The model under review builds one solid part; all positions refer to its coordinate system, in mm. Round coordinates to 2 decimals unless told otherwise and drop trailing zeros. Order: outer loops, then holes, each group sorted by start corner. A loop starts at its lowest first (then second) coordinate and runs counter-clockwise, first axis right, second up. Notation, with made-up numbers: M 59,-8 L 113,-8 A16 ccw 113,18 Z; hole C 73,-29 d3. An arc over 180 degrees is marked long. Answer as a JSON object with one key per item and string values. Group by question number.
1. Add section C-C on y = 1. Give the number of separate pieces and of enclosed holes in the cut face, and give its area (3 significant figures).
2. Add section A-A on z = 0. State the section outline as (x, y) points, and give its area (3 significant figures).
3. Mouldability with a two-part tool opening along X and no side actions: class faces 1 (the face through (9.174, 0.986, 15.343)), 2 (the face through (-0.3, 0, 7.8)), 3 (the face through (-24.14, 1.01, -9.89)) as released by +X, released by -X, zero draft, split by the parting line, or undercut.
4. Add section B-B on x = 0. State the section outline as (y, z) points.
5. Add section D-D on z = 9.5. State the section outline as (x, y) points.
6. Clearance check with flat-ended pins moving along their axes: P1, Ø4, axis at x = 17.87, z = -4.79, coming from the +Y side; P2, Ø2.5, axis at x = -17.87, z = -4.79, coming from the +Y side. State where each tip first meets the part, or that it passes through.
7. To check wall thickness, follow probe 1 along Z at (x, y) = (10.5, 1.1); probe 2 along X at (y, z) = (1.15, -4.75); probe 3 along X at (y, z) = (1.5, -4). State the ranges of each line that lie inside material, in increasing order. Write a range as [from, to].
```python
from build123d import *

# Parameters (mm, degrees)
SKETCH_2_W      = 50
SKETCH_2_H      = 30.788152334
SKETCH_2_R      = 6.75
SKETCH_2_R_2    = 1.45
EXTRUDE_1_DEPTH = 2
FILLET_2_R      = 3


with BuildPart() as part:
    # 草图2 → 凸台-拉伸1 (new body)
    with BuildSketch(Plane(origin=(0, 0, 0), x_dir=(1, 0, 0), z_dir=(0, 1, 0))):
        with Locations((0, -4.605923833)):
            Rectangle(SKETCH_2_W, SKETCH_2_H)
        with Locations(Location((0, 0, 0), (0, 0, 270))):
            Circle(SKETCH_2_R, mode=Mode.SUBTRACT)
        with Locations(Location((-8.227241336, 4.75, 0), (0, 0, 270))):
            Circle(SKETCH_2_R_2, mode=Mode.SUBTRACT)
        with Locations(Location((0, -9.5, 0), (0, 0, 270))):
            Circle(SKETCH_2_R_2, mode=Mode.SUBTRACT)
        with Locations(Location((8.227241336, 4.75, 0), (0, 0, 90))):
            Circle(SKETCH_2_R_2, mode=Mode.SUBTRACT)
        with Locations(Location((-10.611164072, -15.154312819, 0), (0, 0, 270))):
            Circle(SKETCH_2_R_2, mode=Mode.SUBTRACT)
        with Locations(Location((-17.869627786, 4.788152334, 0), (0, 0, 270))):
            Circle(SKETCH_2_R_2, mode=Mode.SUBTRACT)
        with Locations(Location((10.611164072, -15.154312819, 0), (0, 0, 90))):
            Circle(SKETCH_2_R_2, mode=Mode.SUBTRACT)
        with Locations(Location((17.869627786, 4.788152334, 0), (0, 0, 90))):
            Circle(SKETCH_2_R_2, mode=Mode.SUBTRACT)
    extrude(amount=EXTRUDE_1_DEPTH)

    # 圆角2
    fillet_2_edges = [part.edges().sort_by_distance(p)[0] for p in [
        (25, 1, 20),
        (-25, 1, 20),
        (-25, 1, -10.788152334),
        (25, 1, -10.788152334),
    ]]
    fillet(fillet_2_edges, radius=FILLET_2_R)


solid = part.part
```
Recorded:
{
 "1": {"separate pieces": "1", "enclosed holes": "8", "area": "1,340 mm²"},
 "2": {"outline": "M -25,0 L -6.75,0 L -6.75,2 L -25,2 Z; M 6.75,0 L 25,0 L 25,2 L 6.75,2 Z", "area": "73.0 mm²"},
 "3": {"face 1": "undercut", "face 2": "zero draft", "face 3": "released by -X"},
 "4": {"outline": "M 0,-10.79 L 2,-10.79 L 2,-6.75 L 0,-6.75 Z; M 0,6.75 L 2,6.75 L 2,8.05 L 0,8.05 Z; M 0,10.95 L 2,10.95 L 2,20 L 0,20 Z"},
 "5": {"outline": "M -25,0 L -1.45,0 L -1.45,2 L -25,2 Z; M 1.45,0 L 25,0 L 25,2 L 1.45,2 Z"},
 "6": {"P1": "stops at y = 2", "P2": "passes through"},
 "7": {"probe 1": "z = [-10.79, 13.71], [16.6, 20]", "probe 2": "x = [-25, -19.32], [-16.42, -9.68], [-6.78, -4.8], [4.8, 6.78], [9.68, 16.42], [19.32, 25]", "probe 3": "x = [-25, -19.09], [-16.65, -9.47], [-6.99, -5.44], [5.44, 6.99], [9.47, 16.65], [19.09, 25]"}
}
